Read the model definition and answer for the solid it produces. Units are mm, in the model's axes. A direction names the side the tool comes from. Coordinates: 2 decimals unless noted, no trailing zeros. Loops run counter-clockwise (first coordinate to the right, second up) from the corner with the lowest first, then second, coordinate; pieces in that order, holes last. Notation, with made-up numbers: (21, 84.25) -> (26, 84.25) arc R16 cw to (26, 94.25) -> close; hole circle Ø9 at (2, -7.5). An arc over 180 degrees is marked (long way). Answer as a JSON object with one key per item and string values. Group by question number.
Q1. This flat-tipped pin is pushed along its axis until it touches: P1, Ø2, axis at x = -6.36, z = 6.36, coming from the -Y side. Where does it stop, or does it pass through?
Q2. Determine the mould class of faces 1 (the cylindrical face through (6.92, 0.78, -5.3)), 2 (the cylindrical face through (-18.41, 0.78, -11.98)), 3 (the cylindrical face through (15.15, 0.78, 15.11)), 4 (the cylindrical face through (12.071, 0.783, 7.255)) for opening direction Z: released by +Z, released by -Z, zero draft, split by the parting line, or undercut.
Q3. For faces 5 (the flat face through (0, 1, 6.35)), 6 (the flat face through (15.875, 1, 2)), determine the directions among +Z, -Z, +X, -X, +Y, -Y from which every point of the face is accessible in a straight line to the end or side of a thin tool.
Q4. The part is cut by section B-B on z = 8.25. Write down the section's boundary in (x, y) (1 decimal).
Q5. Straight lines are drawn through the part: line 1 along Z through (x, y) = (-15, 1.4) (3 decimals); line 2 along Z through (x, y) = (-3, 1.1) (3 decimals); line 3 along X through (y, z) = (1.5, -7.75) (3 decimals). For each, find the intervals that lie inside material, in ascending order. Write a range as [from, to].
Q6. The part is cut by section D-D on z = -3. Write down the section's boundary in (x, y) (1 decimal), and give its area (3 significant figures).
Q7. The part is cut by section C-C on y = 0.65. State how many separate pieces and enclosed holes the cut face has, and give its area (3 significant figures).
from build123d import *

# Parameters (mm, degrees)
SKETCH1_W           = 31.75
SKETCH1_H           = 25.4
SKETCH1_R           = 7.1374
SKETCH1_R_2         = 1.2
SKETCH1_R_3         = 1.905
BOSS_EXTRUDE1_DEPTH = 1.5875
SKETCH2_W           = 31.75
SKETCH2_H           = 3.175
BOSS_EXTRUDE2_DEPTH = 1.5875
SKETCH5_R           = 1.905
BOSS_EXTRUDE4_DEPTH = 1.5875
SKETCH6_R           = 1.905
CUT_EXTRUDE1_DEPTH  = 2.5875
BOSS_EXTRUDE3_DEPTH = 1.5875
FILLET2_R           = 0.635
FILLET3_R           = 2.54


with BuildPart() as part:
    # Sketch1 → Boss-Extrude1 (new body)
    with BuildSketch(Plane(origin=(0, 0, 0), x_dir=(1, 0, 0), z_dir=(0, 1, 0))):
        Rectangle(SKETCH1_W, SKETCH1_H)
        Circle(SKETCH1_R, mode=Mode.SUBTRACT)
        with Locations((-6.363961031, -6.363961031)):
            Circle(SKETCH1_R_2, mode=Mode.SUBTRACT)
        with Locations((-6.363961031, 6.363961031)):
            Circle(SKETCH1_R_2, mode=Mode.SUBTRACT)
        with Locations((6.363961031, 6.363961031)):
            Circle(SKETCH1_R_2, mode=Mode.SUBTRACT)
        with Locations((6.363961031, -6.363961031)):
            Circle(SKETCH1_R_2, mode=Mode.SUBTRACT)
        with Locations((-12.319, -9.144)):
            Circle(SKETCH1_R_3, mode=Mode.SUBTRACT)
        with Locations((-12.319, 9.144)):
            Circle(SKETCH1_R_3, mode=Mode.SUBTRACT)
        with Locations((12.319, 9.144)):
            Circle(SKETCH1_R_3, mode=Mode.SUBTRACT)
        with Locations((12.319, -9.144)):
            Circle(SKETCH1_R_3, mode=Mode.SUBTRACT)
    extrude(amount=BOSS_EXTRUDE1_DEPTH)

    # Sketch2 → Boss-Extrude2 (add, through all)
    with BuildSketch(Plane(origin=(0, 1.5875, 0), x_dir=(1, 0, 0), z_dir=(0, 1, 0))):
        with Locations((0, -14.2875)):
            Rectangle(SKETCH2_W, SKETCH2_H)
    extrude(amount=-BOSS_EXTRUDE2_DEPTH)

    # Sketch5 → Boss-Extrude4 (add, through all)
    with BuildSketch(Plane(origin=(0, 1.5875, 0), x_dir=(1, 0, 0), z_dir=(0, 1, 0))):
        with Locations((-12.319, 9.144)):
            Circle(SKETCH5_R)
        with Locations((-12.319, -9.144)):
            Circle(SKETCH5_R)
        with BuildLine():
            Line((-19.177, 12.7), (-15.875, 12.7))
            Line((-15.875, 12.7), (-15.875, 4.87211828))
            ThreePointArc((-15.875, 4.87211828), (-16.91465929, 3.175), (-15.875, 1.47788172))
            Line((-15.875, 1.47788172), (-15.875, -15.875))
            Line((-15.875, -15.875), (-19.177, -15.875))
            Line((-19.177, -15.875), (-19.177, 12.7))
        make_face()
    extrude(amount=-BOSS_EXTRUDE4_DEPTH)

    # Sketch6 → Cut-Extrude1 (cut, through all)
    with BuildSketch(Plane(origin=(0, 1.5875, 0), x_dir=(1, 0, 0), z_dir=(0, 1, 0))):
        with Locations((-15.00965929, 3.175)):
            Circle(SKETCH6_R)
    extrude(amount=-CUT_EXTRUDE1_DEPTH, mode=Mode.SUBTRACT)

    # Sketch3 → Boss-Extrude3 (add, through all)
    with BuildSketch(Plane(origin=(0, 1.5875, 0), x_dir=(1, 0, 0), z_dir=(0, 1, 0))):
        with BuildLine():
            Line((-3.258830889, 6.35), (3.258830889, 6.35))
            ThreePointArc((3.258830889, 6.35), (0, 7.1374), (-3.258830889, 6.35))
        make_face()
        with BuildLine():
            Line((3.258830889, -6.35), (-3.258830889, -6.35))
            ThreePointArc((-3.258830889, -6.35), (0, -7.1374), (3.258830889, -6.35))
        make_face()
    extrude(amount=-BOSS_EXTRUDE3_DEPTH)

    # Fillet2
    fillet2_edges = [part.edges().sort_by_distance(p)[0] for p in [
        (-3.258830889, 0.79375, -6.35),
        (3.258830889, 0.79375, -6.35),
        (3.258830889, 0.79375, 6.35),
        (-3.258830889, 0.79375, 6.35),
    ]]
    fillet(fillet2_edges, radius=FILLET2_R)

    # Fillet3
    fillet3_edges = [part.edges().sort_by_distance(p)[0] for p in [
        (15.875, 0.79375, 15.875),
        (-19.177, 0.79375, 15.875),
        (-19.177, 0.79375, -12.7),
        (15.875, 0.79375, -12.7),
    ]]
    fillet(fillet3_edges, radius=FILLET3_R)


solid = part.part
Final values:
{
 "1": {"P1": "passes through"},
 "2": {"face 1": "undercut", "face 2": "released by -Z", "face 3": "released by +Z", "face 4": "undercut"},
 "3": {"face 5": "+Y, -Y", "face 6": "+Z, -Z, +X, +Y, -Y"},
 "4": {"outline": "(-19.2, 0) -> (10.6, 0) -> (10.6, 1.6) -> (-19.2, 1.6) -> close; (14, 0) -> (15.9, 0) -> (15.9, 1.6) -> (14, 1.6) -> close"},
 "5": {"line 1": "z = [-12.7, -5.08], [-1.27, 15.875]", "line 2": "z = [-12.7, -6.35], [6.35, 15.875]", "line 3": "x = [-19.177, 11.021], [13.617, 15.875]"},
 "6": {"outline": "(-19.2, 0) -> (-16.9, 0) -> (-16.9, 1.6) -> (-19.2, 1.6) -> close; (-13.1, 0) -> (-6.5, 0) -> (-6.5, 1.6) -> (-13.1, 1.6) -> close; (6.5, 0) -> (15.9, 0) -> (15.9, 1.6) -> (6.5, 1.6) -> close", "area": "29.1 mm2"},
 "7": {"separate pieces": "1", "enclosed holes": "8", "area": "791 mm2"}
}
